```python
from build123d import *

# Parameters (mm, degrees)
BOSS_EXTRUDE1_DEPTH = 5
SKETCH2_W           = 20
SKETCH2_H           = 5
BOSS_EXTRUDE2_DEPTH = 12


with BuildPart() as part:
    # Sketch1 → Boss-Extrude1 (new body)
    with BuildSketch(Plane.XY):
        with BuildLine():
            ThreePointArc((6, 15), (0, 21), (-6, 15))
            Line((-6, 15), (6, 15))
        make_face()
        with BuildLine():
            Line((6, 15), (-6, 15))
            ThreePointArc((-6, 15), (0, 9), (6, 15))
        make_face()
        with BuildLine():
            ThreePointArc((6, 15), (0, 9), (-6, 15))
            Line((-6, 15), (-6, -15))
            Line((-6, -15), (6, -15))
            Line((6, -15), (6, 15))
        make_face()
    extrude(amount=BOSS_EXTRUDE1_DEPTH)

    # Sketch2 → Boss-Extrude2 (add)
    with BuildSketch(Plane(origin=(6, 0, 0), x_dir=(0, 0, -1), z_dir=(1, 0, 0))):
        with Locations((-15, -12.5)):
            Rectangle(SKETCH2_W, SKETCH2_H)
    extrude(amount=-BOSS_EXTRUDE2_DEPTH)


solid = part.part
```
Work out the finished part from the listing and answer in its coordinate system (mm). A direction names the side the tool comes from. Give positions to 0.01 mm unless a question says otherwise; leave off trailing zeros. Loops run counter-clockwise (first coordinate to the right, second up) from the corner with the lowest first, then second, coordinate; pieces in that order, holes last. Notation, with made-up numbers: (6.25, 14) -> (29.25, 14) arc R23 ccw to (29.25, 37) -> close; hole circle Ø6 at (43.25, 14). An arc over 180 degrees is marked (long way). One line per question, with ' | ' between items. Start each with the question number.
1) For faces 1 (the face through (-6, -4, 4)), 2 (the face through (0, 6, 5)), determine the directions among +Z, -Z, +X, -X, +Y, -Y from which every point of the face is accessible in a straight line to the end or side of a thin tool.
2) Section D-D, the plane x = -3.75 is taken. Determine the outline of the cut face in (y, z), then the cut area to 3 significant figures.
3) Section C-C, the plane y = -1.5 is taken. Determine the outline of the cut face in (x, z).
4) Section B-B, the plane z = 15.25 is taken. Determine the outline of the cut face in (x, y), then the cut area to 3 significant figures.
5) This flat-tipped pin is pushed along its axis until it touches: pin 1 (2 mm diameter, centred on x = 1, z = 21, fed in from +Y). Where does it stop, or does it pass through?
6) Straight lines are drawn through the part: L1, parallel to Z at x = 5, y = 7; L2, parallel to Y at x = -4, z = 7.75; L3, parallel to X at y = 18.5, z = 4.75. For each, find the intervals that lie inside material, in ascending order.
7) Section A-A, the plane x = 0 is taken. Determine the outline of the cut face in (y, z).
Resolved:
1) face 1: +Z, -Z, -X, +Y, -Y | face 2: +Z, +X, -X, +Y
2) outline: (-15, 0) -> (19.68, 0) -> (19.68, 5) -> (-10, 5) -> (-10, 25) -> (-15, 25) -> close | area: 273 mm2
3) outline: (-6, 0) -> (6, 0) -> (6, 5) -> (-6, 5) -> close
4) outline: (-6, -15) -> (6, -15) -> (6, -10) -> (-6, -10) -> close | area: 60.0 mm2
5) pin 1: y = -10
6) L1: 0 to 5 | L2: -15 to -10 | L3: -4.87 to 4.87
7) outline: (-15, 0) -> (21, 0) -> (21, 5) -> (-10, 5) -> (-10, 25) -> (-15, 25) -> close
